from build123d import *

# Parameters (mm, degrees)
SKETCH1_W            = 10
SKETCH1_H            = 10
BOSS_EXTRUDE1_DEPTH  = 2.2
SKETCH2_R            = 0.595
BOSS_EXTRUDE2_DEPTH  = 12.03
LPATTERN1_COUNT      = 4
LPATTERN1_PITCH      = 2.5
LPATTERN1_COUNT_DIR2 = 4
LPATTERN1_PITCH_DIR2 = 2.5


with BuildPart() as part:
    # Sketch1 → Boss-Extrude1 (new body)
    with BuildSketch(Plane(origin=(0, 0, 0), x_dir=(1, 0, 0), z_dir=(0, 1, 0))):
        Rectangle(SKETCH1_W, SKETCH1_H)
    extrude(amount=BOSS_EXTRUDE1_DEPTH)

    # Sketch2 → Boss-Extrude2 (add)
    with BuildSketch(Plane(origin=(0, 2.2, 0), x_dir=(1, 0, 0), z_dir=(0, 1, 0))):
        with Locations(Location((-3.595, -3.685, 0), (0, 0, 90))):
            Circle(SKETCH2_R)
    boss_extrude2 = extrude(amount=BOSS_EXTRUDE2_DEPTH)

    # LPattern1: Boss-Extrude2 4 × 4
    with Locations(*[(i * LPATTERN1_PITCH, 0, -j * LPATTERN1_PITCH_DIR2) for i in range(LPATTERN1_COUNT) for j in range(LPATTERN1_COUNT_DIR2) if (i, j) != (0, 0)]):
        add(boss_extrude2)


solid = part.part
Work out the finished part from the listing and answer in its coordinate system (mm). A direction names the side the tool comes from. Round coordinates to 2 decimals unless told otherwise and drop trailing zeros. Loops run counter-clockwise (first coordinate to the right, second up) from the corner with the lowest first, then second, coordinate; pieces in that order, holes last. Notation, with made-up numbers: (40.5, -5.75) -> (56.5, -5.75) arc R24 cw to (56.5, 7.25) -> close; hole circle Ø11 at (18.5, 20). An arc over 180 degrees is marked (long way). Use one line per item in the form item = value.
(1) Find section A-A on y = 6.75. Give the number of separate pieces and of enclosed holes in the cut face, then the cut area to 3 significant figures.
Answer list:
separate_pieces = 16
enclosed_holes = 0
area = 17.8 mm2
(2) Find section D-D on z = 4. Give the vertices of the cut face in (x, y), then the cut area to 3 significant figures.
Answer list:
outline = (-5, 0) -> (5, 0) -> (5, 2.2) -> (4.41, 2.2) -> (4.41, 14.23) -> (3.4, 14.23) -> (3.4, 2.2) -> (1.91, 2.2) -> (1.91, 14.23) -> (0.9, 14.23) -> (0.9, 2.2) -> (-0.59, 2.2) -> (-0.59, 14.23) -> (-1.6, 14.23) -> (-1.6, 2.2) -> (-3.09, 2.2) -> (-3.09, 14.23) -> (-4.1, 14.23) -> (-4.1, 2.2) -> (-5, 2.2) -> close
area = 70.6 mm2
(3) Flat-ended cylindrical pins translate along their axes: P1, Ø2, axis at y = 5, z = 0, coming from the +X side; P2, Ø1.5, axis at y = 9, z = -0.5, coming from the -X side; P3, Ø6, axis at x = -4, y = 11.5, coming from the +Z side. Find the tip coordinate at first contact, or state that the pin passes through.
Answer list:
P1 = 4.47
P2 = -4.19
P3 = 4.28
(4) A tool of negligible diameter and unlimited length cuts with its end or side. For faces 1 (the cylindrical face through (4.486, 8.131, -3.686)), 2 (the flat face through (4, 14.23, -1)), from which of +Z, -Z, +X, -X, +Y, -Y can it reach the whole face along a straight path? Write none if from no direction.
Answer list:
face_1 = +Y
face_2 = +Z, -Z, +X, -X, +Y
(5) For a pull along X with two mould halves and no side action, classify faces 3 (the flat face through (-3.6, 14.23, 3.7)), 4 (the cylindrical face through (0.815, 8.131, 1.262)), 5 (the flat face through (5, 1, 0)) as released by +X, released by -X, zero draft, split by the parting line, or undercut.
Answer list:
face_3 = zero draft
face_4 = undercut
face_5 = released by +X
(6) Find section B-B on z = 2. Give the vertices of the cut face in (x, y).
Answer list:
outline = (-5, 0) -> (5, 0) -> (5, 2.2) -> (-5, 2.2) -> close
(7) Straight lines are drawn through the part: line 1 (X direction, y = 5, z = -1.25); line 2 (X direction, y = 8.75, z = -1.75); line 3 (Y direction, x = -0.5, z = -2). For each, find the intervals that lie inside material, in ascending order.
Answer list:
line_1 = -4.19 to -3, -1.69 to -0.5, 0.81 to 2, 3.31 to 4.5
line_2 = -4 to -3.19, -1.5 to -0.69, 1 to 1.81, 3.5 to 4.31
line_3 = 0 to 2.2
(8) Find section C-C on x = 1.75. Give the vertices of the cut face in (y, z).
Answer list:
outline = (0, -5) -> (2.2, -5) -> (2.2, -4.3) -> (14.23, -4.3) -> (14.23, -3.33) -> (2.2, -3.33) -> (2.2, -1.8) -> (14.23, -1.8) -> (14.23, -0.83) -> (2.2, -0.83) -> (2.2, 0.7) -> (14.23, 0.7) -> (14.23, 1.67) -> (2.2, 1.67) -> (2.2, 3.2) -> (14.23, 3.2) -> (14.23, 4.17) -> (2.2, 4.17) -> (2.2, 5) -> (0, 5) -> close
